The listing builds one solid part. Answer for the finished solid, in the listing's coordinates (mm). Face numbers are marked on the shaded views. A direction names the side the tool comes from. Round coordinates to 2 decimals unless told otherwise and drop trailing zeros. Write each loop counter-clockwise with the first axis right and the second up, starting at its lowest first coordinate (ties: lowest second). Pieces come first, ordered by that corner, then holes. Notation, with made-up numbers: (46, 63) - (76, 63) arc R21 ccw to (76, 97) - close; hole circle Ø7 at (-39.5, 67). An arc over 180 degrees is marked (long way). Return JSON: item names as keys, results as strings. Group by question number.
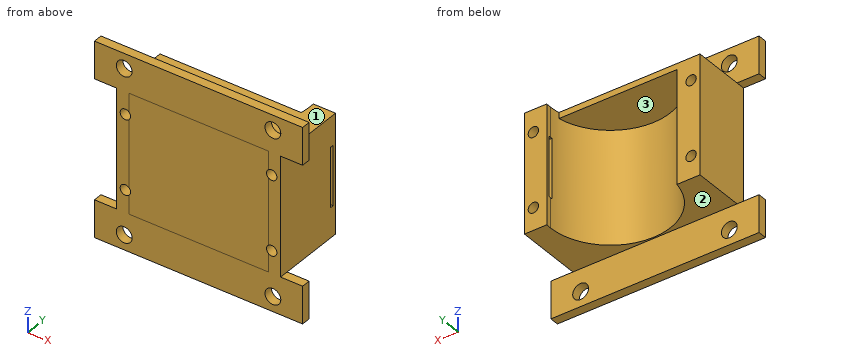
from build123d import *

# Parameters (mm, degrees)
SKETCH1_W                       = 10.823103443
SKETCH1_H                       = 51.052518719
BOSS_EXTRUDE1_DEPTH             = 50.8
SKETCH2_W                       = 177.8
SKETCH2_H                       = 31.75
BOSS_EXTRUDE2_DEPTH             = 7.62
F_1_2_START                     = -59.944
F_1_2_CLEARANCE_HOLE1_OUTLINE_R = 6.74624
F_1_2_CLEARANCE_HOLE1_DEPTH     = 7.62
SKETCH7_W                       = 140.208
SKETCH7_H                       = 43.432518719
BOSS_EXTRUDE3_DEPTH             = 5.08
CUT_EXTRUDE1_REACH              = 190.918
CUT_EXTRUDE1_END_RADIUS         = 51.203999954
SKETCH6_W                       = 50.8
SKETCH6_H                       = 3.474999908
SKETCH8_R                       = 4.4323
CUT_EXTRUDE2_DEPTH              = 138.353334223
SKETCH9_R                       = 4.4323
CUT_EXTRUDE3_DEPTH              = 132.62094122


# Read off the part's stored shape, not the designer's step: 1/2 Clearance Hole1
with BuildPart() as part:
    # Sketch1 → Boss-Extrude1 (new, symmetric)
    with BuildSketch(Plane.XY):
        with Locations((-64.692448278, -34.41774064)):
            Rectangle(SKETCH1_W, SKETCH1_H)
        with BuildLine():
            ThreePointArc((-2e-09, -59.944), (-39.117081832, -45.421768404), (-59.280896557, -8.891481281))
            Line((-59.280896557, -8.891481281), (-59.280896557, -59.944))
            Line((-59.280896557, -59.944), (-2e-09, -59.944))
        make_face()
        with BuildLine():
            Line((-50.42609614, -8.891481281), (-59.280896557, -8.891481281))
            ThreePointArc((-59.280896557, -8.891481281), (-39.117081832, -45.421768404), (-2e-09, -59.944))
            ThreePointArc((-2e-09, -59.944), (42.386808891, -42.386808892), (59.944, 0))
            ThreePointArc((59.944, 0), (59.902397652, 2.232911009), (59.777648353, 4.462722648))
            Line((59.777648353, 4.462722648), (51.009153275, 4.462722648))
            ThreePointArc((51.009153275, 4.462722648), (51.155265092, 2.233487109), (51.203999954, 0))
            ThreePointArc((51.203999954, 0), (4.462722648, -51.009153275), (-50.42609614, -8.891481281))
        make_face()
        with BuildLine():
            ThreePointArc((59.944, 0), (42.386808891, -42.386808892), (-2e-09, -59.944))
            Line((-2e-09, -59.944), (59.944, -59.944))
            Line((59.944, -59.944), (59.944, 0))
        make_face()
        with BuildLine():
            Line((70.104, 4.462722648), (59.777648353, 4.462722648))
            ThreePointArc((59.777648353, 4.462722648), (59.902397652, 2.232911009), (59.944, 0))
            Line((59.944, 0), (59.944, -59.944))
            Line((59.944, -59.944), (70.104, -59.944))
            Line((70.104, -59.944), (70.104, 4.462722648))
        make_face()
    extrude(amount=BOSS_EXTRUDE1_DEPTH, both=True)

    # Sketch2 → Boss-Extrude2 (add)
    with BuildSketch(Plane.XZ.offset(59.944)):
        with Locations((0, 66.675)):
            Rectangle(SKETCH2_W, SKETCH2_H)
    boss_extrude2 = extrude(amount=-BOSS_EXTRUDE2_DEPTH)

    # 1/2 Clearance Hole1 outline → 1/2 Clearance Hole1 (cut)
    with BuildSketch(Plane(origin=(0, 0, 0), x_dir=(1, 0, 0), z_dir=(0, 1, 0)).offset(F_1_2_START)):
        with Locations((63.5, -69.85)):
            Circle(F_1_2_CLEARANCE_HOLE1_OUTLINE_R)
        with Locations((-63.5, -69.85)):
            Circle(F_1_2_CLEARANCE_HOLE1_OUTLINE_R)
    f_1_2_clearance_hole1 = extrude(amount=F_1_2_CLEARANCE_HOLE1_DEPTH, mode=Mode.SUBTRACT)

    # Mirror1: Boss-Extrude2, 1/2 Clearance Hole1 across plane
    add(boss_extrude2.mirror(Plane.XY))
    add(f_1_2_clearance_hole1.mirror(Plane.XY), mode=Mode.SUBTRACT)

    # Sketch7 → Boss-Extrude3 (add)
    with BuildSketch(Plane.XY.offset(50.8)):
        with Locations((0, -30.607740641)):
            Rectangle(SKETCH7_W, SKETCH7_H)
    extrude(amount=-BOSS_EXTRUDE3_DEPTH)

    # Cut-Extrude1: up to this cylinder (the profile starts outside it)
    cut_extrude1_end = Plane(origin=(0, 0, 0), z_dir=(0, 0, 1)) * Cylinder(CUT_EXTRUDE1_END_RADIUS, 485.243999908, mode=Mode.PRIVATE)
    # Sketch6 → Cut-Extrude1 (cut, up to the surface)
    with BuildSketch(Plane(origin=(70.104, 0, 0), x_dir=(0, 0, -1), z_dir=(1, 0, 0)), mode=Mode.PRIVATE) as cut_extrude1_sk1:
        Rectangle(SKETCH6_W, SKETCH6_H)
    cut_extrude1_tool1 = extrude(cut_extrude1_sk1.sketch, amount=-CUT_EXTRUDE1_REACH, mode=Mode.PRIVATE) - cut_extrude1_end
    add(cut_extrude1_tool1.solids().sort_by_distance((70.104, 0, 0))[0], mode=Mode.SUBTRACT)

    # Sketch8 → Cut-Extrude2 (cut, through all)
    with BuildSketch(Plane(origin=(0, 4.462722648, 0), x_dir=(1, 0, 0), z_dir=(0, 1, 0))):
        with Locations(Location((62.484, 31.75, 0), (0, 0, 180))):
            Circle(SKETCH8_R)
        with Locations(Location((62.484, -31.75, 0), (0, 0, 180))):
            Circle(SKETCH8_R)
    extrude(amount=-CUT_EXTRUDE2_DEPTH, mode=Mode.SUBTRACT)

    # Sketch9 → Cut-Extrude3 (cut, through all)
    with BuildSketch(Plane(origin=(0, -8.891481281, 0), x_dir=(1, 0, 0), z_dir=(0, 1, 0))):
        with Locations(Location((-62.484, 31.75, 0), (0, 0, 270))):
            Circle(SKETCH9_R)
        with Locations(Location((-62.484, -31.75, 0), (0, 0, 270))):
            Circle(SKETCH9_R)
    extrude(amount=-CUT_EXTRUDE3_DEPTH, mode=Mode.SUBTRACT)


solid = part.part
(1) Consider line 1 (X direction, y = -56.25, z = 69.85); line 2 (Z direction, x = 63, y = -54); line 3 (X direction, y = -26, z = 31.75). Determine where each line is inside the solid, lowest interval first.
(2) For the marked faces 1, 2 and 3, determine the directions among +Z, -Z, +X, -X, +Y, -Y from which every point of the face is accessible in a straight line to the end or side of a thin tool.
(3) Flat-ended cylindrical pins translate along their axes: pin 1 (10 mm diameter, centred on x = 5.5, z = 23, fed in from +Y); pin 2 (7 mm diameter, centred on x = 62.484, z = 31.75, fed in from -Y); pin 3 (8 mm diameter, centred on x = 22.5, z = -25.5, fed in from +Y); pin 4 (3 mm diameter, centred on x = 66.5, y = -29.5, fed in from +Z). Find the tip coordinate at first contact, or state that the pin passes through.
(4) Find section A-A (z = 22). Write down the section's boundary in (x, y).
(5) Find section B-B (z = 69.85). Write down the section's boundary in (x, y), plus the area to 3 significant figures.
(6) Find section D-D (x = 32.5). Write down the section's boundary in (y, z), plus the area to 3 significant figures.
(7) Find section C-C (y = -24). Write down the section's boundary in (x, z), plus the area to 3 significant figures.
Check sheet entries:
{
 "1": {"line 1": "x = -88.9 to -70.25, -56.75 to 56.75, 70.25 to 88.9", "line 2": "z = -82.55 to -76.58, -63.12 to -36.15, -27.35 to 27.35, 36.15 to 63.12, 76.58 to 82.55", "line 3": "x = -70.1 to -66.92, -58.05 to -44.11, 44.11 to 58.05, 66.92 to 70.1"},
 "2": {"face 1": "+Z, +X, -X, +Y", "face 2": "-Z, +X, -X, +Y", "face 3": "-Z, +Y"},
 "3": {"pin 1": "stops at y = -50.12", "pin 2": "passes through", "pin 3": "stops at y = -43.81", "pin 4": "stops at z = 50.8"},
 "4": {"outline": "(-70.1, -59.94) - (70.1, -59.94) - (70.1, -1.74) - (51.17, -1.74) arc R51.2 cw to (-50.43, -8.89) - (-70.1, -8.89) - close; (51.01, 4.46) arc R51.2 cw to (51.17, 1.74) - (70.1, 1.74) - (70.1, 4.46) - close"},
 "5": {"outline": "(-88.9, -59.94) - (-70.25, -59.94) - (-70.25, -52.32) - (-88.9, -52.32) - close; (-56.75, -59.94) - (56.75, -59.94) - (56.75, -52.32) - (-56.75, -52.32) - close; (70.25, -59.94) - (88.9, -59.94) - (88.9, -52.32) - (70.25, -52.32) - close", "area": "1,150 mm^2"},
 "6": {"outline": "(-59.94, -82.55) - (-52.32, -82.55) - (-52.32, -50.8) - (-39.57, -50.8) - (-39.57, 45.72) - (-8.89, 45.72) - (-8.89, 50.8) - (-52.32, 50.8) - (-52.32, 82.55) - (-59.94, 82.55) - close", "area": "2,710 mm^2"},
 "7": {"outline": "(-70.1, -50.8) - (-45.23, -50.8) - (-45.23, 45.72) - (45.23, 45.72) - (45.23, -50.8) - (70.1, -50.8) - (70.1, 50.8) - (-70.1, 50.8) - close; hole circle Ø8.86 at (-62.48, -31.75); hole circle Ø8.86 at (-62.48, 31.75); hole circle Ø8.86 at (62.48, -31.75); hole circle Ø8.86 at (62.48, 31.75)", "area": "5,270 mm^2"}
}
